Read the model definition and answer for the solid it produces. Units are mm, in the model's axes. Face numbers are marked on the shaded views. A direction names the side the tool comes from. Round coordinates to 2 decimals unless told otherwise and drop trailing zeros. Write each loop counter-clockwise with the first axis right and the second up, starting at its lowest first coordinate (ties: lowest second). Pieces come first, ordered by that corner, then holes. Notation, with made-up numbers: (88, -29) - (97, -29) arc R7 ccw to (97, -17) - close; hole circle Ø3 at (-12.5, 51). An arc over 180 degrees is marked (long way). One line per item, written item: value. Start each with the question number.
(1) Find the intervals of material crossed by L1, parallel to Y at x = 6.75, z = 7.5; L2, parallel to Z at x = 13, y = 40; L3, parallel to X at y = 41, z = 1.65, in increasing order.
(2) A cutting plane is placed at D-D, the plane x = 14.5. Determine the outline of the cut face in (y, z).
(3) For the marked faces 1 and 2, determine the directions among +Z, -Z, +X, -X, +Y, -Y from which every point of the face is accessible in a straight line to the end or side of a thin tool.
(4) A cutting plane is placed at C-C, the plane y = 22. Determine the outline of the cut face in (x, z), plus the area to 3 significant figures.
(5) A cutting plane is placed at A-A, the plane z = 1.5. Determine the outline of the cut face in (x, y), plus the area to 3 significant figures.
(6) A cutting plane is placed at B-B, the plane y = 41.5. State how many separate pieces and enclosed holes the cut face has, plus the area to 3 significant figures.
(7) Flat-ended cylindrical pins translate along their axes: pin 1 Ø1.2 at (x, z) = (4.5, 6) entering from +Y; pin 2 Ø3 at (x, y) = (19, 41.5) entering from -Z (1 decimal); pin 3 Ø1.3 at (y, z) = (3.5, 6.5) entering from -X; pin 4 Ø5 at (y, z) = (3.5, 7.5) entering from +X. Find the tip coordinate at first contact, or state that the pin passes through.
Autodesk Inventor part; units mm, degrees
ref_plane "YZ Plane" through (0, 0, 0) normal (1, 0, 0) x (0, 1, 0)
ref_plane "XZ Plane" through (0, 0, 0) normal (0, 1, 0) x (-1, 0, 0)
ref_plane "XY Plane" through (0, 0, 0) normal (0, 0, 1) x (1, 0, 0)
sketch "Skizze1" plane through (0, 0, 0) normal (0, 0, 1) x (1, 0, 0)
  line L0 (10, 0) -> (23, 38.5)
  line L1 (23, 38.5) -> (23, 44.5)
  line L2 (23, 44.5) -> (0, 44.5)
  line L3 (0, 44.5) -> (0, 0)
  line L4 (10, 0) -> (0, 0)
  dimension "d0" = 38.5
  dimension "d1" = 6
  dimension "d2" = 23
  dimension "d4" = 10
extrude "Extrusion1" add sketch "Skizze1" along normal blind 5
sketch "Skizze3" plane through (0, 0, 5) normal (0, 0, 1) x (1, 0, 0)
  line L0 (23, 38.5) -> (23, 44.5)
  line L1 (23, 41.5) -> (18.9958, 41.5) construction
  line L2 (4.0042, 41) -> (0, 41) construction
  line L3 (0, 44.5) -> (0, 0) construction
  dimension "d35" = 0.5
  dimension "d36" = 15
hole "Bohrung2" at (4.0042, 41, 5) at (18.9958, 41.5, 5) direction (0, 0, -1) diameter 3.5 end through all
sketch "Skizze4" plane through (0, 0, 5) normal (0, 0, 1) x (1, 0, 0)
  line L0 (0, 44.5) -> (0, 0)
  line L1 (0, 9) -> (13.039, 9)
  line L2 (0, 0) -> (10, 0)
  line L3 (10, 0) -> (23, 38.5)
  dimension "d24" = 9
extrude "Extrusion2" add sketch "Skizze4" along normal blind 5.5
sketch "Skizze2" plane through (0, 0, 0) normal (-1, 0, 0) x (0, 0, 1)
  line L0 (0, 0) -> (5, 0)
  line L1 (5, 9) -> (10.5, 9)
  line L2 (10.5, 9) -> (10.5, 0)
  point P0 (7.5, 3.5)
  dimension "d27" = 3.5
  dimension "d37" = 3
hole "Bohrung1" at (0, 3.5, 7.5) direction (1, 0, 0) diameter 4.3 depth 8
fillet "Rundung2" radius 8 1 edges at (5, 0, 0)
fillet "Rundung3" radius 3 1 edges at (6.5195, 9, 10.5)
fillet "Rundung4" radius 3 1 edges at (5, 0, 10.5)
chamfer "Fasen1" distance 1 angle 45 2 edges at (4.0042, 42.75, 5) (18.9958, 43.25, 5)
fillet "Rundung5" radius 2 2 edges at (0, 44.5, 2.5) (23, 44.5, 2.5)
properties part number "Lupfer Seite"
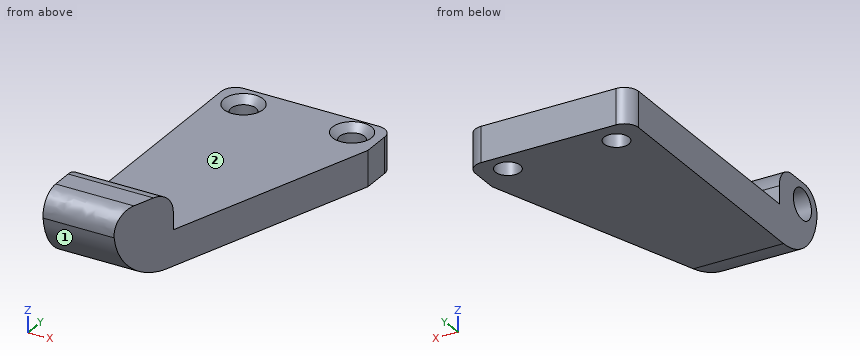
Here are the results:
1. L1: 0.03 to 1.35, 5.65 to 9
1. L2: 0 to 5
1. L3: 0 to 2.25, 5.75 to 17.32, 20.67 to 23
2. outline: (13.33, 0) - (44.5, 0) - (44.5, 5) - (13.33, 5) - close
3. face 1: -Z, +X, -X, -Y
3. face 2: +Z, +X, -X, +Y
4. outline: (0, 0) - (17.43, 0) - (17.43, 5) - (0, 5) - close
4. area: 87.1 mm²
5. outline: (0, 3.34) - (11.13, 3.34) - (23, 38.5) - (23, 42.5) arc R2 ccw to (21, 44.5) - (2, 44.5) arc R2 ccw to (0, 42.5) - close; hole circle Ø3.5 at (4, 41); hole circle Ø3.5 at (19, 41.5)
5. area: 717 mm²
6. separate pieces: 3
6. enclosed holes: 0
6. area: 78.7 mm²
7. pin 1: y = 9
7. pin 2: through
7. pin 3: x = 8
7. pin 4: x = 12.03
